Source: three-view drawing plus pictorial views. Frame: mm from the lowest corner of the part. Round coordinates to 2 decimals unless told otherwise and drop trailing zeros. Loops run counter-clockwise (first coordinate to the right, second up) from the corner with the lowest first, then second, coordinate; pieces in that order, holes last. Notation, with made-up numbers: (-19, -21.75) -> (6, -21.75) arc R35 ccw to (6, 17.25) -> close; hole circle Ø5 at (60.5, 67). An arc over 180 degrees is marked (long way). Return JSON: item names as keys, results as strings. Group by question number.
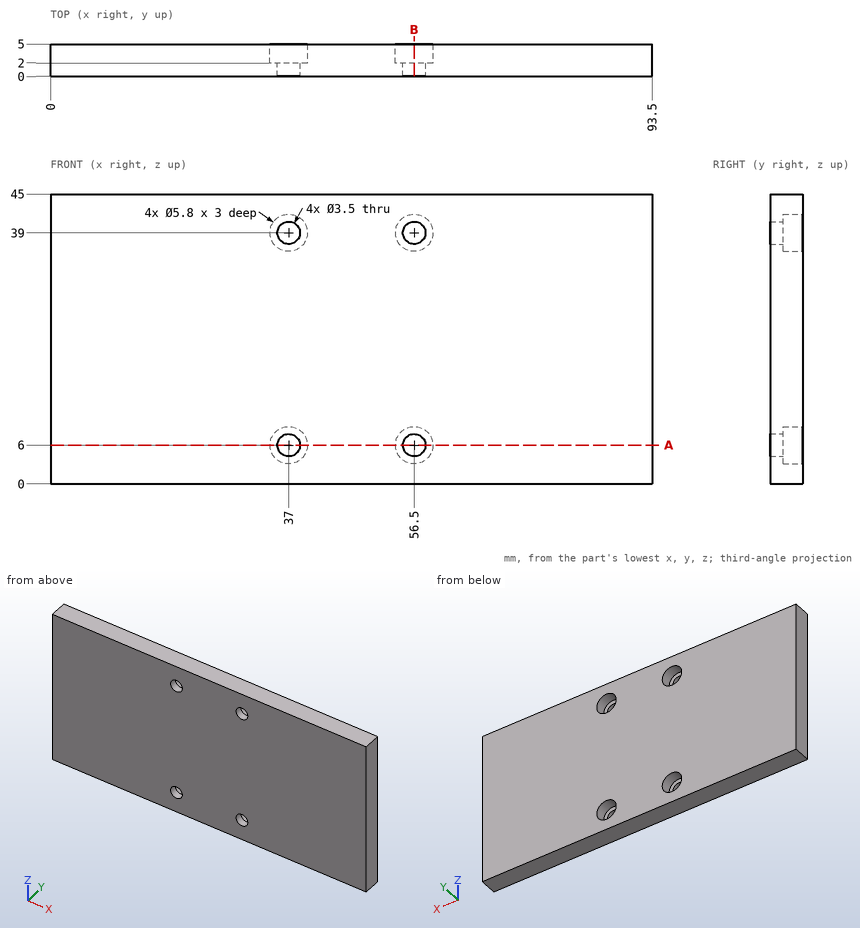
(1) Cut plane A-A (z = 6). Return loops of the section in (x, y).
(2) Cut plane B-B (x = 56.5). Return loops of the section in (y, z).
(3) Pin query (flat end, axial travel): pin 1 (5.5 mm diameter, centred on x = 56.5, z = 39, fed in from +Y). Return the tip coordinate at first contact, or that it passes through.
(4) Ray query, line 1 (X direction, y = 2.8, z = 39); line 2 (Z direction, x = 56.5, y = 3.4); line 3 (X direction, y = 0.7, z = 6). Return the intervals inside material, ascending.
Answers follow:
{
 "1": {"outline": "(0, 0) -> (35.25, 0) -> (35.25, 2) -> (34.1, 2) -> (34.1, 5) -> (0, 5) -> close; (38.75, 0) -> (54.75, 0) -> (54.75, 2) -> (53.6, 2) -> (53.6, 5) -> (39.9, 5) -> (39.9, 2) -> (38.75, 2) -> close; (58.25, 0) -> (93.5, 0) -> (93.5, 5) -> (59.4, 5) -> (59.4, 2) -> (58.25, 2) -> close"},
 "2": {"outline": "(0, 0) -> (5, 0) -> (5, 3.1) -> (2, 3.1) -> (2, 4.25) -> (0, 4.25) -> close; (0, 7.75) -> (2, 7.75) -> (2, 8.9) -> (5, 8.9) -> (5, 36.1) -> (2, 36.1) -> (2, 37.25) -> (0, 37.25) -> close; (0, 40.75) -> (2, 40.75) -> (2, 41.9) -> (5, 41.9) -> (5, 45) -> (0, 45) -> close"},
 "3": {"pin 1": "y = 2"},
 "4": {"line 1": "0 to 34.1, 39.9 to 53.6, 59.4 to 93.5", "line 2": "0 to 3.1, 8.9 to 36.1, 41.9 to 45", "line 3": "0 to 35.25, 38.75 to 54.75, 58.25 to 93.5"}
}
